Design review of the part shown in the three views and the two pictorial views. Dimensions are in mm from the part's minimum x, y and z. A direction names the side the tool comes from. Give positions to 0.01 mm unless a question says otherwise; leave off trailing zeros. Order: outer loops, then holes, each group sorted by start corner. A loop starts at its lowest first (then second) coordinate and runs counter-clockwise, first axis right, second up.
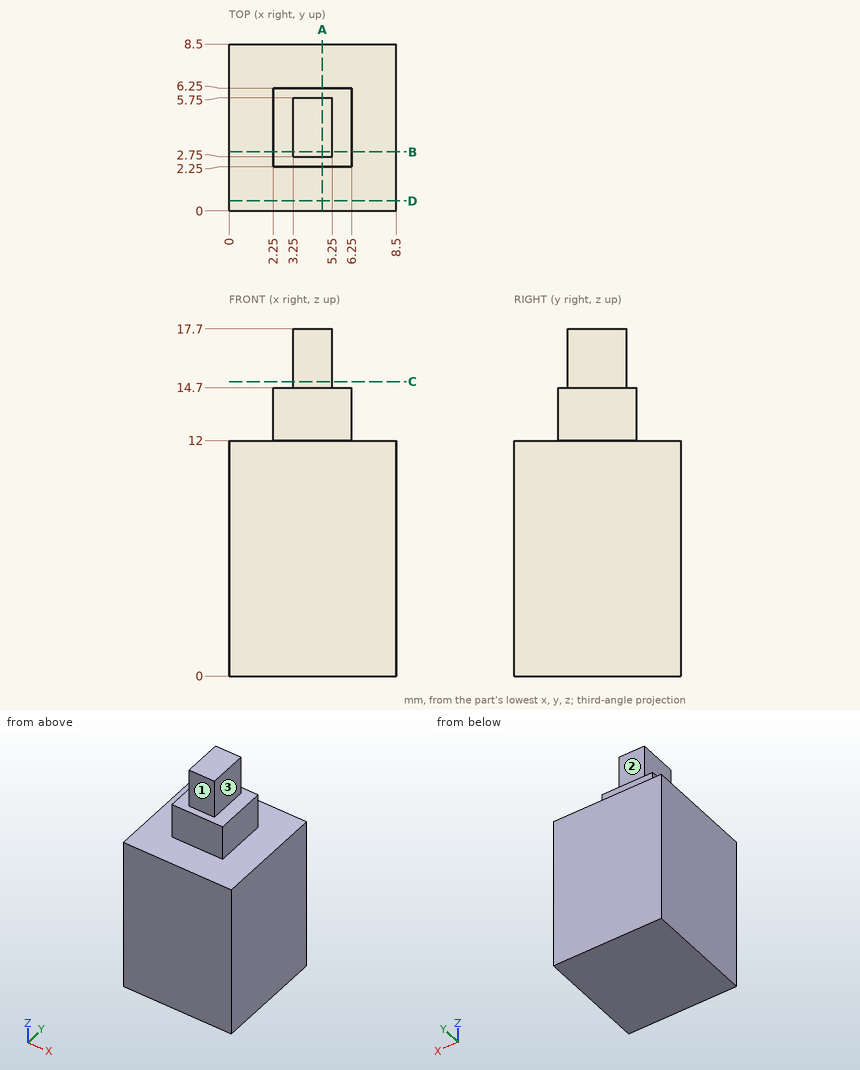
Item 1: Take a section at D-D (y = 0.5). Give the boundary of the cut face in (x, z), and give its area (3 significant figures).
Values found:
outline: (0, 0) - (8.5, 0) - (8.5, 12) - (0, 12) - close
area: 102 mm2
Item 2: Take a section at B-B (y = 3). Give the boundary of the cut face in (x, z), and give its area (3 significant figures).
Values found:
outline: (0, 0) - (8.5, 0) - (8.5, 12) - (6.25, 12) - (6.25, 14.7) - (5.25, 14.7) - (5.25, 17.7) - (3.25, 17.7) - (3.25, 14.7) - (2.25, 14.7) - (2.25, 12) - (0, 12) - close
area: 119 mm2
Item 3: Take a section at A-A (x = 4.75). Give the boundary of the cut face in (y, z), and give its area (3 significant figures).
Values found:
outline: (0, 0) - (8.5, 0) - (8.5, 12) - (6.25, 12) - (6.25, 14.7) - (5.75, 14.7) - (5.75, 17.7) - (2.75, 17.7) - (2.75, 14.7) - (2.25, 14.7) - (2.25, 12) - (0, 12) - close
area: 122 mm2
Item 4: Take a section at C-C (z = 15). Give the boundary of the cut face in (x, y), and give its area (3 significant figures).
Values found:
outline: (3.25, 2.75) - (5.25, 2.75) - (5.25, 5.75) - (3.25, 5.75) - close
area: 6.00 mm2
Item 5: For line 1 (Z direction, x = 4.25, y = 2.5); line 2 (X direction, y = 5.25, z = 14); line 3 (Z direction, x = 4.5, y = 1.5), list the stretches that pass through material, from the lowest coordinate up.
Values found:
line 1: z = 0 to 14.7
line 2: x = 2.25 to 6.25
line 3: z = 0 to 12
Item 6: Clearance check with flat-ended pins moving along their axes: pin 1 Ø2 at (x, z) = (6, 2.5) entering from -Y; pin 2 Ø1 at (x, y) = (3.5, 6.5) entering from +Z; pin 3 Ø0.6 at (x, z) = (4.5, 16) entering from +Y; pin 4 Ø1.3 at (x, z) = (5, 14) entering from -Y. State where each tip first meets the part, or that it passes through.
Values found:
pin 1: stops at y = 0
pin 2: stops at z = 14.7
pin 3: stops at y = 5.75
pin 4: stops at y = 2.25
Item 7: For the marked faces 1, 2 and 3, list the 3-axis set-ups (+Z, -Z, +X, -X, +Y, -Y) from which the entire face can be reached by the end or side of a thin tool; tool diameter is ignored.
Values found:
face 1: +Z, +X, -X, -Y
face 2: +Z, +X, -X, +Y
face 3: +Z, +X, +Y, -Y
